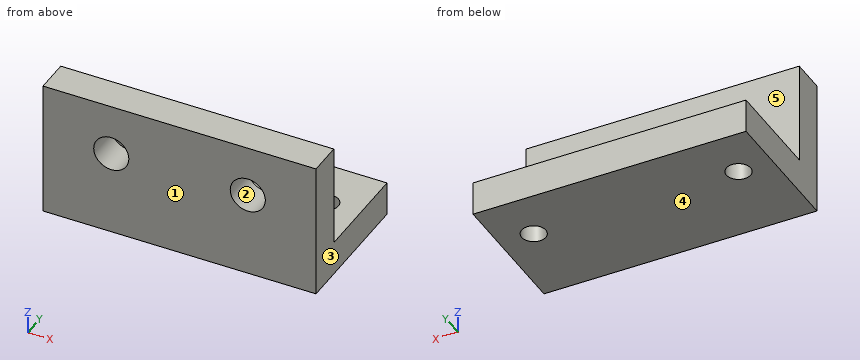
from build123d import *

# Parameters (mm, degrees)
BOSS_EXTRUDE1_DEPTH       = 25.4
F_1_4_CLEARANCE_HOLE1_D   = 6.5278
F_8_CLEARANCE_HOLE1_D     = 4.4958
F_8_CLEARANCE_HOLE1_DEPTH = 6.35
F_8_CLEARANCE_HOLE1_TIP   = 1.350674586


with BuildPart() as part:
    # Sketch1 → Boss-Extrude1 (new, symmetric)
    with BuildSketch(Plane(origin=(0, 0, 0), x_dir=(0, 0, -1), z_dir=(1, 0, 0))):
        Polygon((0, 0), (0, 25.4), (-6.35, 25.4), (-6.35, 6.35), (-25.4, 6.35), (-25.4, 0), align=None)
    extrude(amount=BOSS_EXTRUDE1_DEPTH, both=True)

    # 1/4 Clearance Hole1 (through all)
    with Locations(Plane(origin=(0, 6.35, 0), x_dir=(1, 0, 0), z_dir=(0, 1, 0))):
        with Locations((-12.7, -15.875), (12.7, -15.875)):
            Hole(F_1_4_CLEARANCE_HOLE1_D / 2)

    # #8 Clearance Hole1
    with Locations(Plane.XY.offset(6.35)):
        with Locations((-19.05, 15.875), (19.05, 15.875)):
            Hole(F_8_CLEARANCE_HOLE1_D / 2, depth=F_8_CLEARANCE_HOLE1_DEPTH)
            with Locations((0, 0, -(F_8_CLEARANCE_HOLE1_DEPTH + F_8_CLEARANCE_HOLE1_TIP / 2))):  # 118° drill point
                Cone(0, F_8_CLEARANCE_HOLE1_D / 2, F_8_CLEARANCE_HOLE1_TIP, mode=Mode.SUBTRACT)


solid = part.part
Check sheet for the modelled part. Datum: model origin and axes. Units: mm. Face numbers are marked on the shaded views. A direction names the side the tool comes from. Give positions to 0.01 mm unless a question says otherwise; leave off trailing zeros. Write each loop counter-clockwise with the first axis right and the second up, starting at its lowest first coordinate (ties: lowest second). Pieces come first, ordered by that corner, then holes. Notation, with made-up numbers: (21.5, 39.25) -> (53.5, 39.25) arc R16 cw to (53.5, 70.25) -> close; hole circle Ø1 at (63, 47). An arc over 180 degrees is marked (long way). One line per item, written item: value. Start each with the question number.
Item 1: Gauge pin test, flat ends, axial feed: pin 1 (4 mm diameter, centred on x = 14, z = 17, fed in from +Y); pin 2 (6 mm diameter, centred on x = -12.7, z = 15.875, fed in from +Y). Record the tip position at first contact, or that the pin passes through.
Item 2: Material ranges on probe 1 along Y at (x, z) = (19.05, 4.75); probe 2 along X at (y, z) = (4.75, 14); probe 3 along Z at (x, y) = (0, 12), recorded low to high. Write a range as from..to.
Item 3: Draft check along X on the marked faces 1, 2 and 3. Enter one of: +X half, -X half, draft (parallel to the pull), parting line (faces both ways), or undercut.
Item 4: Tool access check on the marked faces 4 and 5. Record the directions out of +Z, -Z, +X, -X, +Y, -Y that give a thin tool (end or side, any length) a straight path to the whole face; none if there is none.
Item 5: Section check C-C on y = 10.75. Record the cut outline in (x, z), then the cut area to 3 significant figures.
Item 6: Section check A-A on x = 12.7. Record the cut outline in (y, z), then the cut area to 3 significant figures.
Item 7: Section check B-B on x = 19.05. Record the cut outline in (y, z).
Item 8: Section check D-D on x = -7. Record the cut outline in (y, z), then the cut area to 3 significant figures.
Results list:
1. pin 1: y = 6.35
1. pin 2: through
2. probe 1: 0..13.63, 18.12..25.4
2. probe 2: -25.4..-15.37, -10.03..10.03, 15.37..25.4
2. probe 3: 0..6.35
3. face 1: draft
3. face 2: undercut
3. face 3: +X half
4. face 4: -Z, +X, -X, +Y, -Y
4. face 5: +Z, +X, -X, +Y
5. outline: (-25.4, 0) -> (25.4, 0) -> (25.4, 6.35) -> (-25.4, 6.35) -> close
5. area: 323 mm²
6. outline: (0, 0) -> (25.4, 0) -> (25.4, 6.35) -> (6.35, 6.35) -> (6.35, 12.61) -> (0, 12.61) -> close; (0, 19.14) -> (6.35, 19.14) -> (6.35, 25.4) -> (0, 25.4) -> close
6. area: 241 mm²
7. outline: (0, 0) -> (13.63, 0) -> (13.63, 6.35) -> (6.35, 6.35) -> (6.35, 25.4) -> (0, 25.4) -> close; (18.12, 0) -> (25.4, 0) -> (25.4, 6.35) -> (18.12, 6.35) -> close
8. outline: (0, 0) -> (25.4, 0) -> (25.4, 6.35) -> (6.35, 6.35) -> (6.35, 25.4) -> (0, 25.4) -> close
8. area: 282 mm²
